CAD build for the part. Positions are in the model's coordinates, mm. A direction names the side the tool comes from. Give positions to 0.01 mm unless a question says otherwise; leave off trailing zeros. Write each loop counter-clockwise with the first axis right and the second up, starting at its lowest first coordinate (ties: lowest second). Pieces come first, ordered by that corner, then holes. Notation, with made-up numbers: (24, -24.5) - (33, -24.5) arc R10 cw to (33, -6.5) - close; hole circle Ø7 at (10, 44). An arc over 180 degrees is marked (long way). Put each result on its own line as item: value. Start each with the question number.
1. Tool access for faces 1 (the cylindrical face through (2.711, 93.996, -9.633)), 2 (the flat face through (75.6, 321, -9)), 3 (the cylindrical face through (2.804, 67.911, -9.633)): list every direction of +Z, -Z, +X, -X, +Y, -Y with a clear straight run to the whole face (end or side of a thin tool).
2. Cut at B-B on z = -6.25. Give the number of separate pieces and of enclosed holes in the cut face, and give its area (3 significant figures).
3. Mould opens along Y. For faces 4 (the cylindrical face through (73.796, 97.511, -9.633)), 5 (the flat face through (38, 285.8, -9)), 6 (the flat face through (112, 178, 0)) say: +Y half, -Y half, draft (parallel to the pull), parting line (faces both ways), or undercut.
4. Drop flat-ended pins along their axis: pin 1 (10 mm diameter, centred on y = 39.5, z = -14, fed in from -X); pin 2 (1.5 mm diameter, centred on x = 63.5, z = -10, fed in from -Y); pin 3 (5.5 mm diameter, centred on x = 46, z = -13.5, fed in from +Y). Give the stop position or say it passes through.
5. Cut at A-A on x = 38. List the corners of the cut face in (y, z).
6. Wall check: line 1 (Y direction, x = 23, z = -10.25); line 2 (X direction, y = 331, z = -5.5); line 3 (Y direction, x = 160, z = -9.5). Give the ranges that are in metal, low to high.
from build123d import *

# Parameters (mm, degrees)
PAD014_DEPTH    = 19
FILLET002_R     = 20
FILLET003_R     = 6
SKETCH029_R     = 2
POCKET019_DEPTH = 19.001


with BuildPart() as part:
    # Sketch017 → Pad014 (new body)
    with BuildSketch(Plane.XY):
        Polygon((275, 216.2), (379.498932, 216.2), (379.498932, -133.8), (275, -133.8), (275, -68.6), (200.4, -68.6), (200.4, -39), (275, -39), (275, 26.4), (200.4, 26.4), (200.4, 56), (275, 56), (275, 121.4), (200.4, 121.4), (200.4, 151), (275, 151), align=None)
    extrude(amount=-PAD014_DEPTH)

    # Fillet002
    fillet002_edges = [part.edges().sort_by_distance(p)[0] for p in [
        (379.498932, 216.2, -9.5),
        (379.498932, -133.8, -9.5),
    ]]
    fillet(fillet002_edges, radius=FILLET002_R)

    # Fillet003
    fillet003_edges = [part.edges().sort_by_distance(p)[0] for p in [
        (200.4, 151, -9.5),
        (200.4, 121.4, -9.5),
        (200.4, 26.4, -9.5),
        (200.4, 56, -9.5),
        (200.4, -39, -9.5),
        (200.4, -68.6, -9.5),
        (275, 151, -9.5),
        (275, 121.4, -9.5),
        (275, 26.4, -9.5),
        (275, -68.6, -9.5),
        (275, -39, -9.5),
        (275, 56, -9.5),
    ]]
    fillet(fillet003_edges, radius=FILLET003_R)

    # Sketch029 (on Face32 of Fillet003) → Pocket019 (cut, through all)
    with BuildSketch(Plane(origin=(0, 0, -19), x_dir=(1, 0, 0), z_dir=(0, 0, -1))):
        with Locations((359.498932, 113.8)):
            Circle(SKETCH029_R)
        with Locations((359.498932, -196.2)):
            Circle(SKETCH029_R)
    extrude(amount=-POCKET019_DEPTH, mode=Mode.SUBTRACT)


with BuildPart() as part_1:
    # Body010 placement: moved
    add(part.part.moved(Location((0, 0, -9))))


with BuildPart() as part_2:
    # Clone placement: moved
    add(part_1.part.moved(Location((-199.4, 134.8, 9))))


solid = part_2.part
Report:
1. face 1: +Z, -Z, -X
1. face 2: +Z, -Z, -X, +Y
1. face 3: +Z, -Z, -X, -Y
2. separate pieces: 1
2. enclosed holes: 2
2. area: 43,000 mm²
3. face 4: undercut
3. face 5: +Y half
3. face 6: draft
4. pin 1: stops at x = 75.6
4. pin 2: stops at y = 66.2
4. pin 3: stops at y = 285.8
5. outline: (66.2, -19) - (95.8, -19) - (95.8, 0) - (66.2, 0) - close; (161.2, -19) - (190.8, -19) - (190.8, 0) - (161.2, 0) - close; (256.2, -19) - (285.8, -19) - (285.8, 0) - (256.2, 0) - close
6. line 1: y = 66.2 to 95.8, 161.2 to 190.8, 256.2 to 285.8
6. line 2: x = 75.6 to 158.1, 162.1 to 180.1
6. line 3: y = 1 to 19, 23 to 329, 333 to 351
